Can you work these out from the model? Positions are in its coordinate system, mm. A direction names the side the tool comes from. Give positions to 0.01 mm unless a question says otherwise; leave off trailing zeros. Order: outer loops, then holes, each group sorted by start corner. A loop starts at its lowest first (then second) coordinate and runs counter-clockwise, first axis right, second up. Notation, with made-up numbers: (43, 80.5) - (97, 80.5) arc R21 ccw to (97, 90.5) - close; hole circle Ø8 at (74.5, -26). An arc over 180 degrees is marked (long way). One line per question, with ' | ' between items.
```python
from build123d import *

# Parameters (mm, degrees)
BOSS_EXTRUDE1_DEPTH      = 58.5
BOSS_EXTRUDE1_DEPTH_BACK = 58.5
SKETCH2_R                = 3.15
CUT_EXTRUDE1_DEPTH       = 58.5
FILLET1_R                = 0.5
CUT_EXTRUDE2_DEPTH       = 3
LPATTERN1_COUNT          = 2
LPATTERN1_PITCH          = 60
FILLET2_R                = 0.5
CUT_EXTRUDE3_DEPTH       = 13.88331
CUT_EXTRUDE3_DEPTH_BACK  = 9.68331


with BuildPart() as part:
    # Sketch1 → Boss-Extrude1 (new, two sides: drawn at the far end of the back side and taken through both)
    with BuildSketch(Plane.XY.offset(-BOSS_EXTRUDE1_DEPTH_BACK)):
        with BuildLine():
            Line((-40, -2.5), (40, -2.5))
            Line((40, -2.5), (40, 2.5))
            Line((40, 2.5), (11.3, 2.5))
            ThreePointArc((11.3, 2.5), (9.249747468, 7.449747468), (4.3, 9.5))
            Line((4.3, 9.5), (2.1, 9.5))
            Line((2.1, 9.5), (2.1, 6))
            Line((2.1, 6), (4.3, 6))
            Line((4.3, 6), (4.3, 2.5))
            Line((4.3, 2.5), (-4.3, 2.5))
            Line((-4.3, 2.5), (-4.3, 6))
            Line((-4.3, 6), (-2.1, 6))
            Line((-2.1, 6), (-2.1, 9.5))
            Line((-2.1, 9.5), (-4.3, 9.5))
            ThreePointArc((-4.3, 9.5), (-9.249747468, 7.449747468), (-11.3, 2.5))
            Line((-11.3, 2.5), (-40, 2.5))
            Line((-40, 2.5), (-40, -2.5))
        make_face()
    extrude(amount=BOSS_EXTRUDE1_DEPTH + BOSS_EXTRUDE1_DEPTH_BACK)

    # Sketch2 → Cut-Extrude1 (cut)
    with BuildSketch(Plane.XZ.offset(2.5)):
        with Locations(Location((-30, 48, 0), (0, 0, 270))):
            Circle(SKETCH2_R)
        with Locations(Location((30, 48, 0), (0, 0, 270))):
            Circle(SKETCH2_R)
        with Locations(Location((30, -48, 0), (0, 0, 270))):
            Circle(SKETCH2_R)
        with Locations(Location((-30, -48, 0), (0, 0, 270))):
            Circle(SKETCH2_R)
    extrude(amount=-CUT_EXTRUDE1_DEPTH, mode=Mode.SUBTRACT)

    # Fillet1
    fillet1_edges = [part.edges().sort_by_distance(p)[0] for p in [
        (-2.1, 7.75, -58.5),
        (-3.2, 9.5, -58.5),
        (-9.249747468, 7.449747468, -58.5),
        (-25.65, 2.5, -58.5),
        (-4.3, 2.5, 0),
        (4.3, 2.5, 0),
        (4.3, 6, 0),
        (2.1, 6, 0),
        (2.1, 9.5, 0),
        (11.3, 2.5, 0),
        (40, 2.5, 0),
        (40, -2.5, 0),
        (-40, -2.5, 0),
        (-40, 2.5, 0),
        (-11.3, 2.5, 0),
        (-2.1, 9.5, 0),
        (-2.1, 6, 0),
        (-4.3, 6, 0),
        (-40, 0, -58.5),
        (0, -2.5, -58.5),
        (40, 0, -58.5),
        (-3.2, 9.5, 58.5),
        (-25.65, 2.5, 58.5),
        (25.65, 2.5, -58.5),
        (-40, 0, 58.5),
        (25.65, 2.5, 58.5),
        (9.249747468, 7.449747468, 58.5),
        (2.1, 7.75, 58.5),
        (3.2, 6, 58.5),
        (4.3, 4.25, 58.5),
        (0, 2.5, 58.5),
        (9.249747468, 7.449747468, -58.5),
        (-4.3, 4.25, 58.5),
        (-3.2, 6, 58.5),
        (-2.1, 7.75, 58.5),
        (-9.249747468, 7.449747468, 58.5),
        (0, -2.5, 58.5),
        (40, 0, 58.5),
        (3.2, 9.5, 58.5),
        (3.2, 9.5, -58.5),
        (-4.3, 4.25, -58.5),
        (2.1, 7.75, -58.5),
        (3.2, 6, -58.5),
        (4.3, 4.25, -58.5),
        (0, 2.5, -58.5),
        (-30, 2.5, 51.15),
        (30, 2.5, -44.85),
        (-30, 2.5, -44.85),
        (30, 2.5, 51.15),
        (-3.2, 6, -58.5),
    ]]
    fillet(fillet1_edges, radius=FILLET1_R)

    # Sketch3 → Cut-Extrude2 (cut)
    with BuildSketch(Plane(origin=(0, 2.5, 0), x_dir=(1, 0, 0), z_dir=(0, 1, 0))):
        Polygon((-24.226497308, 48), (-27.113248654, 53), (-32.886751346, 53), (-35.773502692, 48), (-32.886751346, 43), (-27.113248654, 43), align=None)
        Polygon((-24.226497308, -48), (-27.113248654, -43), (-32.886751346, -43), (-35.773502692, -48), (-32.886751346, -53), (-27.113248654, -53), align=None)
    cut_extrude2 = extrude(amount=-CUT_EXTRUDE2_DEPTH, mode=Mode.SUBTRACT)

    # LPattern1: Cut-Extrude2 ×2
    with Locations(*[(i * LPATTERN1_PITCH, 0, 0) for i in range(1, LPATTERN1_COUNT)]):
        add(cut_extrude2, mode=Mode.SUBTRACT)

    # Fillet2
    fillet2_edges = [part.edges().sort_by_distance(p)[0] for p in [
        (-25.669872981, 2.5, -45.5),
        (-25.669872981, 2.5, -50.5),
        (-30, 2.5, -53),
        (-34.330127019, 2.5, -50.5),
        (-34.330127019, 2.5, -45.5),
        (-30, 2.5, -43),
        (-25.669872981, 2.5, 50.5),
        (-25.669872981, 2.5, 45.5),
        (-30, 2.5, 43),
        (-34.330127019, 2.5, 45.5),
        (-34.330127019, 2.5, 50.5),
        (-30, 2.5, 53),
        (34.330127019, 2.5, -45.5),
        (34.330127019, 2.5, -50.5),
        (30, 2.5, -53),
        (25.669872981, 2.5, -50.5),
        (25.669872981, 2.5, -45.5),
        (30, 2.5, -43),
        (34.330127019, 2.5, 50.5),
        (34.330127019, 2.5, 45.5),
        (30, 2.5, 43),
        (25.669872981, 2.5, 45.5),
        (25.669872981, 2.5, 50.5),
        (30, 2.5, 53),
    ]]
    fillet(fillet2_edges, radius=FILLET2_R)

    # Sketch6 → Cut-Extrude3 (cut, two sides: drawn at the far end of the back side and taken through both)
    with BuildSketch(Plane.ZY.offset(-2.1).offset(-CUT_EXTRUDE3_DEPTH_BACK)):
        Polygon((47.07, 9.5), (58.5, -3.2), (58.5, 9.5), align=None)
    extrude(amount=CUT_EXTRUDE3_DEPTH + CUT_EXTRUDE3_DEPTH_BACK, mode=Mode.SUBTRACT)


solid = part.part
```
(1) If I drill on line 1 (X direction, y = -1.65, z = -48); line 2 (Z direction, x = 33, y = 0.25); line 3 (Y direction, x = -3, z = -7.5), over which ranges is the centre line in solid material (lowest first)?
Answer below:
line 1: -40 to -33.15, -26.85 to 26.85, 33.15 to 40 | line 2: -58.5 to -52.8, -43.2 to 43.2, 52.8 to 58.5 | line 3: -2.5 to 2.5, 6 to 9.5
(2) Imagine slicing it at A-A (x = -30). List the corners of the cut face in (y, z) for me, and give its area (3 significant figures).
Answer below:
outline: (-2.5, -58) arc R0.5 ccw to (-2, -58.5) - (2, -58.5) arc R0.5 ccw to (2.5, -58) - (2.5, -53.5) arc R0.5 ccw to (2, -53) - (-0.5, -53) - (-0.5, -51.15) - (-2.5, -51.15) - close; (-2.5, -44.85) - (-0.5, -44.85) - (-0.5, -43) - (2, -43) arc R0.5 ccw to (2.5, -42.5) - (2.5, 42.5) arc R0.5 ccw to (2, 43) - (-0.5, 43) - (-0.5, 44.85) - (-2.5, 44.85) - close; (-2.5, 51.15) - (-0.5, 51.15) - (-0.5, 53) - (2, 53) arc R0.5 ccw to (2.5, 53.5) - (2.5, 58) arc R0.5 ccw to (2, 58.5) - (-2, 58.5) arc R0.5 ccw to (-2.5, 58) - close | area: 499 mm^2
(3) Will these pins go through, and if not, where does the flat tip stop? pin 1 (0.8 mm diameter, centred on y = 4, z = -23.5, fed in from +X); pin 2 (8 mm diameter, centred on x = -33, z = -48.5, fed in from +Y); pin 3 (10 mm diameter, centred on x = -11, z = 41.5, fed in from +Y); pin 4 (5 mm diameter, centred on x = 30, z = -48, fed in from +Y).
Answer below:
pin 1: x = 11.21 | pin 2: y = 2.5 | pin 3: y = 9.29 | pin 4: through
(4) Imagine slicing it at C-C (x = 22). List the corners of the cut face in (y, z) for me, and give its area (3 significant figures).
Answer below:
outline: (-2.5, -58) arc R0.5 ccw to (-2, -58.5) - (2, -58.5) arc R0.5 ccw to (2.5, -58) - (2.5, 58) arc R0.5 ccw to (2, 58.5) - (-2, 58.5) arc R0.5 ccw to (-2.5, 58) - close | area: 585 mm^2
(5) On a 3-axis mill with a long thin cutter (end or side, diameter ignored), from which of +Z, -Z, +X, -X, +Y, -Y can I reach the whole of each face in a straight line? I mean faces 5 (the face through (26, 2.5, -1)), 6 (the face through (2.1, 8, -5)), 7 (the face through (-25.52, 2.35, 50.53)). Say none if no direction works.
Answer below:
face 5: +Z, -Z, +X, +Y | face 6: +Z, -Z, +Y | face 7: +Y
(6) If we mould it in two halves opening along Z, with no side actions, what happens to faces 1 (the face through (32.5, -0.5, 50.2)), 2 (the face through (-9.03, 7.66, -3.3)), 3 (the face through (25, 0, 58.5)), 4 (the face through (25.69, 0.768, -50.535))? For each: released by +Z, released by -Z, zero draft, split by the parting line, or undercut.
Answer below:
face 1: undercut | face 2: zero draft | face 3: released by +Z | face 4: undercut
